from build123d import *

# Parameters (mm, degrees)
SKETCH8_R               = 2.55
CUT_EXTRUDE1_DEPTH      = 8.5
CUT_EXTRUDE1_TAPER      = 1
SKETCH9_R               = 1.5
CUT_EXTRUDE2_DEPTH      = 2
CUT_EXTRUDE5_DEPTH      = 3
CUT_EXTRUDE5_DEPTH_BACK = 10.6000001


with BuildPart() as part:
    # Sketch1 → Revolve1 (revolve)
    with BuildSketch(Plane.XY):
        with BuildLine():
            Line((0, 45.78749956), (2.45, 45.78749956))
            Line((2.45, 45.78749956), (2.45, 43.78749956))
            Line((2.45, 43.78749956), (3.5, 43.78749956))
            ThreePointArc((3.5, 43.78749956), (4.560660172, 43.348159732), (5, 42.28749956))
            Line((5, 42.28749956), (5, 36.78749956))
            ThreePointArc((5, 36.78749956), (4.560660172, 35.726839388), (3.5, 35.28749956))
            Line((3.5, 35.28749956), (3.5, 34.18749956))
            Line((3.5, 34.18749956), (0, 34.18749956))
            Line((0, 34.18749956), (0, 45.78749956))
        make_face()
    revolve(axis=Axis((0, 45.78749956, 0), (0, -1, 0)))

    # Sketch8 → Cut-Extrude1 (cut)
    with BuildSketch(Plane.XZ.offset(-34.18749956)):
        Circle(SKETCH8_R)
    extrude(amount=-CUT_EXTRUDE1_DEPTH, taper=CUT_EXTRUDE1_TAPER, mode=Mode.SUBTRACT)

    # Sketch9 → Cut-Extrude2 (cut)
    with BuildSketch(Plane(origin=(0, 45.78749956, 0), x_dir=(1, 0, 0), z_dir=(0, 1, 0))):
        Circle(SKETCH9_R)
    extrude(amount=-CUT_EXTRUDE2_DEPTH, mode=Mode.SUBTRACT)

    # Sketch10 → Cut-Extrude5 (cut, two sides)
    with BuildSketch(Plane(origin=(0, 43.78749956, 0), x_dir=(1, 0, 0), z_dir=(0, 1, 0))) as cut_extrude5_sk:
        with BuildLine():
            Line((-0.4, 0.349856808), (-0.4, 1.445683229))
            ThreePointArc((-0.4, 1.445683229), (-1.271196067, 0.796279197), (-1.475320312, -0.270979664))
            Line((-1.475320312, -0.270979664), (-0.4, 0.349856808))
        make_face()
        with BuildLine():
            ThreePointArc((1.5, 0), (1.193733639, 0.908295106), (0.4, 1.445683229))
            Line((0.4, 1.445683229), (0.4, 0.349856808))
            Line((0.4, 0.349856808), (1.475320312, -0.270979664))
            ThreePointArc((1.475320312, -0.270979664), (1.493817336, -0.136050602), (1.5, 0))
        make_face()
        with BuildLine():
            Line((0, -0.342963515), (-1.124809572, -0.992372625))
            ThreePointArc((-1.124809572, -0.992372625), (0, -1.5), (1.124809572, -0.992372625))
            Line((1.124809572, -0.992372625), (0, -0.342963515))
        make_face()
    extrude(amount=CUT_EXTRUDE5_DEPTH, mode=Mode.SUBTRACT)
    extrude(cut_extrude5_sk.sketch, amount=-CUT_EXTRUDE5_DEPTH_BACK, mode=Mode.SUBTRACT)


solid = part.part
Read the model definition and answer for the solid it produces. Units are mm, in the model's axes. A direction names the side the tool comes from. Give positions to 0.01 mm unless a question says otherwise; leave off trailing zeros. Write each loop counter-clockwise with the first axis right and the second up, starting at its lowest first coordinate (ties: lowest second). Pieces come first, ordered by that corner, then holes. Notation, with made-up numbers: (76.5, -18) - (116.5, -18) arc R18 cw to (116.5, 1) - close; hole circle Ø9 at (33.5, 42.25). An arc over 180 degrees is marked (long way). Use CSV: the item, a comma, the result in double quotes. Start each with the question number.
(1) Find section B-B (y = 39.5). Give the vertices of the cut face in (x, z).
(2) For faces 5 (the flat face through (0, 42.687, 0)), 6 (the flat face through (-0.945, 43.245, -0.035)), 7 (the flat face through (-2, 43.787, -2)), determine the directions among +Z, -Z, +X, -X, +Y, -Y from which every point of the face is accessible in a straight line to the end or side of a thin tool.
(3) Find section A-A (y = 36). Give the vertices of the cut face in (x, z).
(4) Determine the mould class of faces 1 (the flat face through (0.57, 43.25, 0.67)), 2 (the flat face through (0, 43.787, 0)), 3 (the cylindrical face through (3.233, 34.73, -1.341)), 4 (the flat face through (0, 45.787, -2)) for opening direction X: +X half, -X half, draft (parallel to the pull), parting line (faces both ways), or undercut.
(5) Consider line 1 along Z through (x, y) = (0, 44.85); line 2 along Z through (x, y) = (0, 40); line 3 along Y through (x, z) = (-1, 2.5). Determine where each line is inside the solid, lowest interval first.
(6) Given P1, Ø0.5, axis at y = 43.5, z = -1, coming from the +X side; P2, Ø2.5, axis at x = 1, z = -0.5, coming from the -Y side; P3, Ø0.9, axis at y = 43, z = -1, coming from the -X side, each flat-ended and moving along its own axis, determine where each tip first touches the part or whether it passes through.
Findings below:
1,outline,"circle Ø10 at (0, 0); hole circle Ø4.91 at (0, 0)"
2,face 5,"-Y"
2,face 6,"+Y, -Y"
2,face 7,"+Y"
3,outline,"circle Ø9.55 at (0, 0); hole circle Ø5.04 at (0, 0)"
4,face 1,"undercut"
4,face 2,"undercut"
4,face 3,"parting line"
4,face 4,"draft"
5,line 1,"-2.45 to -1.5, 1.5 to 2.45"
5,line 2,"-5 to -2.45, 2.45 to 5"
5,line 3,"34.19 to 43.79"
6,P1,"x = 4.55"
6,P2,"y = 42.69"
6,P3,"x = -4.9"
